Work out the finished part from the listing and answer in its coordinate system (mm). A direction names the side the tool comes from. Round coordinates to 2 decimals unless told otherwise and drop trailing zeros. Write each loop counter-clockwise with the first axis right and the second up, starting at its lowest first coordinate (ties: lowest second). Pieces come first, ordered by that corner, then holes.
from build123d import *

# Parameters (mm, degrees)
F0_R     = 3.5
F1_DEPTH = 5
F2_R     = 9.99999
F4_START = 5
F3_W     = 5
F3_H     = 20
F4_DEPTH = 95
F5_R     = 3.5
F6_DEPTH = 79.3
F7_R     = 9.99999
F8_DEPTH = 16.5
F3_W_2   = 7
F9_DEPTH = 10
F10_SIZE = 6.99999


# Not quite as in the source:
# - a fillet or chamfer is up to 0.001 mm smaller than in the source, because OpenCascade refuses the exact size


with BuildPart() as f1:
    # F0 (on Top) → F1 (new body)
    with BuildSketch(Plane.XY):
        with BuildLine():
            Line((-36.1016022205, 30.0462352857), (-46.2016022205, 30.0462352857))
            Line((-46.2016022205, 30.0462352857), (-46.2016022205, 10.0462352857))
            Line((-46.2016022205, 10.0462352857), (-36.1016022205, 10.0462352857))
            ThreePointArc((-36.1016022205, 10.0462352857), (-46.1016022205, 20.0462352857), (-36.1016022205, 30.0462352857))
        make_face()
        with BuildLine():
            Line((53.7983977795, 30.0462352857), (-36.1016022205, 30.0462352857))
            ThreePointArc((-36.1016022205, 30.0462352857), (-29.0305344087, 27.1173030976), (-26.1016022205, 20.0462352857))
            ThreePointArc((-26.1016022205, 20.0462352857), (-29.0305344087, 12.9751674738), (-36.1016022205, 10.0462352857))
            Line((-36.1016022205, 10.0462352857), (53.7983977795, 10.0462352857))
            Line((53.7983977795, 10.0462352857), (53.7983977795, 30.0462352857))
        make_face()
        with BuildLine():
            ThreePointArc((-26.1016022205, 20.0462352857), (-29.0305344087, 27.1173030976), (-36.1016022205, 30.0462352857))
            ThreePointArc((-36.1016022205, 30.0462352857), (-46.1016022205, 20.0462352857), (-36.1016022205, 10.0462352857))
            ThreePointArc((-36.1016022205, 10.0462352857), (-29.0305344087, 12.9751674738), (-26.1016022205, 20.0462352857))
        make_face()
        with Locations((-36.1016022205, 20.0462352857)):
            Circle(F0_R, mode=Mode.SUBTRACT)
    extrude(amount=F1_DEPTH)

    # F2 (radius 10 in the source; OpenCascade refuses exactly that, so slightly less here)
    f2_edges = [f1.edges().sort_by_distance(p)[0] for p in [
        (-46.201602, 30.046235, 2.5),
        (-46.201602, 10.046235, 2.5),
    ]]
    fillet(f2_edges, radius=F2_R)

    # F3 (on Top) → F4 (join)
    with BuildSketch(Plane.XY.offset(F4_START)):
        with Locations((51.2983977795, 20.0760087371)):
            Rectangle(F3_W, F3_H)
    extrude(amount=F4_DEPTH)

    # F5 (on Right) → F6 (cut)
    with BuildSketch(Plane.YZ):
        with Locations((20.0534593314, 89.2638255358)):
            Circle(F5_R)
    extrude(amount=F6_DEPTH, mode=Mode.SUBTRACT)

    # F7 (radius 10 in the source; OpenCascade refuses exactly that, so slightly less here)
    f7_edges = [f1.edges().sort_by_distance(p)[0] for p in [
        (51.298398, 10.076009, 100),
        (51.298398, 30.076009, 100),
    ]]
    fillet(f7_edges, radius=F7_R)

    # F0 (on Top) → F8 (join)
    with BuildSketch(Plane.XY):
        with BuildLine():
            ThreePointArc((-26.1016022205, 20.0462352857), (-29.0305344087, 27.1173030976), (-36.1016022205, 30.0462352857))
            ThreePointArc((-36.1016022205, 30.0462352857), (-46.1016022205, 20.0462352857), (-36.1016022205, 10.0462352857))
            ThreePointArc((-36.1016022205, 10.0462352857), (-29.0305344087, 12.9751674738), (-26.1016022205, 20.0462352857))
        make_face()
        with Locations((-36.1016022205, 20.0462352857)):
            Circle(F0_R, mode=Mode.SUBTRACT)
    extrude(amount=F8_DEPTH)

    # F3 (on Top) → F9 (join)
    with BuildSketch(Plane.XY):
        with Locations((51.2983977795, 20.0760087371)):
            Rectangle(F3_W, F3_H)
        with Locations((45.2983977795, 20.0760087371)):
            Rectangle(F3_W_2, F3_H)
    extrude(amount=F9_DEPTH)

    # F10 (size 7 in the source; OpenCascade refuses exactly that, so slightly less here)
    f10_edges = [f1.edges().sort_by_distance(p)[0] for p in [
        (41.798398, 20.076009, 10),
    ]]
    chamfer(f10_edges, length=F10_SIZE)


solid = f1.part
Q1. Find section B-B (y = 18). Count the separate pieces of the cut face and the enclosed holes in it, plus the area to 3 significant figures.
Q2. A tool of negligible diameter and unlimited length cuts with its end or side. For faces 5 (the face through (8, 10.046, 2)), 6 (the face through (-32, 20, 16.5)), from which of +Z, -Z, +X, -X, +Y, -Y can it reach the whole face along a straight path? Write none if from no direction.
Q3. Find the intervals of material crossed by L1, parallel to Z at x = -12, y = 12; L2, parallel to X at y = 29, z = 56.5; L3, parallel to X at y = 27, z = 13, in increasing order.
Q4. Find section A-A (z = 14). Determine the outline of the cut face in (x, y), plus the area to 3 significant figures.
Q5. The mould has two halves that part along Y. Classify faces 1 (the face through (8, 20, 5)), 2 (the face through (51.263, 21.935, 92.215)), 3 (the face through (4, 30.046, 2)), 4 (the face through (51.333, 12.928, 96.993)): +Y half, -Y half, draft (parallel to the pull), parting line (faces both ways), or undercut.
Q6. Given pin 1 (5 mm diameter, centred on x = -40, y = 21.5, fed in from +Z); pin 2 (1.5 mm diameter, centred on y = 14.5, z = 78.5, fed in from -X); pin 3 (5 mm diameter, centred on x = 51.5, z = 48.5, fed in from -Y), each flat-ended and moving along its own axis, determine where each tip first touches the part or whether it passes through.
Report:
1. separate pieces: 3
1. enclosed holes: 0
1. area: 1,090 mm2
2. face 5: +Z, -Z, +X, -X, -Y
2. face 6: +Z, -X, +Y, -Y
3. L1: z = 0 to 5
3. L2: x = 48.8 to 53.8
3. L3: x = -43.29 to -28.92, 48.8 to 53.8
4. outline: circle Ø20 at (-36.1, 20.05); (48.8, 10.08) - (53.8, 10.08) - (53.8, 30.08) - (48.8, 30.08) - close; hole circle Ø7 at (-36.1, 20.05)
4. area: 376 mm2
5. face 1: draft
5. face 2: undercut
5. face 3: +Y half
5. face 4: -Y half
6. pin 1: stops at z = 16.5
6. pin 2: stops at x = 48.8
6. pin 3: stops at y = 10.08
